Read the model definition and answer for the solid it produces. Units are mm, in the model's axes. Face numbers are marked on the shaded views. A direction names the side the tool comes from. Give positions to 0.01 mm unless a question says otherwise; leave off trailing zeros. Loops run counter-clockwise (first coordinate to the right, second up) from the corner with the lowest first, then second, coordinate; pieces in that order, holes last. Notation, with made-up numbers: (30, 54.5) -> (69, 54.5) arc R28 ccw to (69, 93.5) -> close; hole circle Ø3 at (45.5, -8.5). An arc over 180 degrees is marked (long way). Write each question's results on one line, items separated by ' | '. Start each with the question number.
Item 1: Find the intervals of material crossed by line 1 (Z direction, x = 1.75, y = 12); line 2 (Y direction, x = -2, z = 2.75); line 3 (X direction, y = 4.5, z = 3.75), in increasing order.
Item 2: Section D-D on x = -1.75 is taken. Write down the section's boundary in (y, z), and give its area (3 significant figures).
Item 3: Determine the mould class of the marked faces 1, 2 and 3 for opening direction Y: +Y half, -Y half, draft (parallel to the pull), parting line (faces both ways), or undercut.
Item 4: Which of the six approach directions +Z, -Z, +X, -X, +Y, -Y give full straight-line access (tool end or side, diameter ignored) to the marked faces 4 and 5?
Item 5: Each of these flat-tipped pins is pushed along its axis until it touches: P1, Ø1, axis at x = 2.5, z = 8, coming from the +Y side; P2, Ø0.5, axis at y = 5.5, z = 3, coming from the +X side; P3, Ø1.7, axis at y = 4.5, z = 8.5, coming from the +X side; P4, Ø0.8, axis at x = -1, y = -14, coming from the -Z side. Where does it stop, or does it pass through?
Item 6: Section A-A on z = 2 is taken. State how many separate pieces and enclosed holes the cut face has, and give its area (3 significant figures).
```python
from build123d import *

# Parameters (mm, degrees)
F0_W     = 7.9375
F0_H     = 35.433
F1_DEPTH = 11.1125
F3_DEPTH = 35.433
F4_R     = 1.35255
F5_DEPTH = 4.7625
F6_R     = 3.175


with BuildPart() as f1:
    # F0 (on Top) → F1 (new body)
    with BuildSketch(Plane.XY):
        Rectangle(F0_W, F0_H)
    extrude(amount=F1_DEPTH)

    # F2 (on face) → F3 (cut, through all)
    with BuildSketch(Plane.XZ.offset(17.7165)):
        Polygon((3.96875, 9.525), (2.38125, 9.525), (2.38125, 8.73125), (1.5875, 8.73125), (1.5875, 7.14375), (2.38125, 7.14375), (2.38125, 6.35), (3.96875, 6.35), align=None)
        Polygon((3.96875, 4.7625), (2.38125, 4.7625), (2.38125, 3.96875), (1.5875, 3.96875), (1.5875, 2.38125), (2.38125, 2.38125), (2.38125, 1.5875), (3.96875, 1.5875), align=None)
    extrude(amount=-F3_DEPTH, mode=Mode.SUBTRACT)

    # F4 (on face) → F5 (cut)
    with BuildSketch(Plane(origin=(0, 0, 0), x_dir=(1, 0, 0), z_dir=(0, 0, -1))):
        with Locations((-0.79375, 14.5415)):
            Circle(F4_R)
        with Locations((-0.79375, -14.5415)):
            Circle(F4_R)
    extrude(amount=-F5_DEPTH, mode=Mode.SUBTRACT)

    # F6
    f6_edges = [f1.edges().sort_by_distance(p)[0] for p in [
        (-3.96875, 17.7165, 5.55625),
        (-3.96875, -17.7165, 5.55625),
    ]]
    fillet(f6_edges, radius=F6_R)


solid = f1.part
```
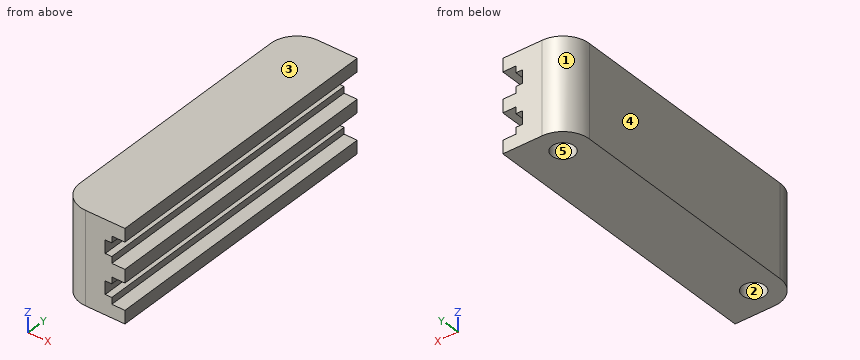
Findings:
1) line 1: 0 to 2.38, 3.97 to 7.14, 8.73 to 11.11 | line 2: -17.48 to -15.15, -13.93 to 13.93, 15.15 to 17.48 | line 3: -3.97 to 1.59
2) outline: (-17.57, 0) -> (-15.5, 0) -> (-15.5, 4.76) -> (-13.58, 4.76) -> (-13.58, 0) -> (13.58, 0) -> (13.58, 4.76) -> (15.5, 4.76) -> (15.5, 0) -> (17.57, 0) -> (17.57, 11.11) -> (-17.57, 11.11) -> close | area: 372 mm2
3) face 1: +Y half | face 2: undercut | face 3: draft
4) face 4: +Z, -Z, -X, +Y, -Y | face 5: -Z
5) P1: through | P2: x = 1.59 | P3: x = 2.38 | P4: z = 4.76
6) separate pieces: 1 | enclosed holes: 2 | area: 209 mm2
